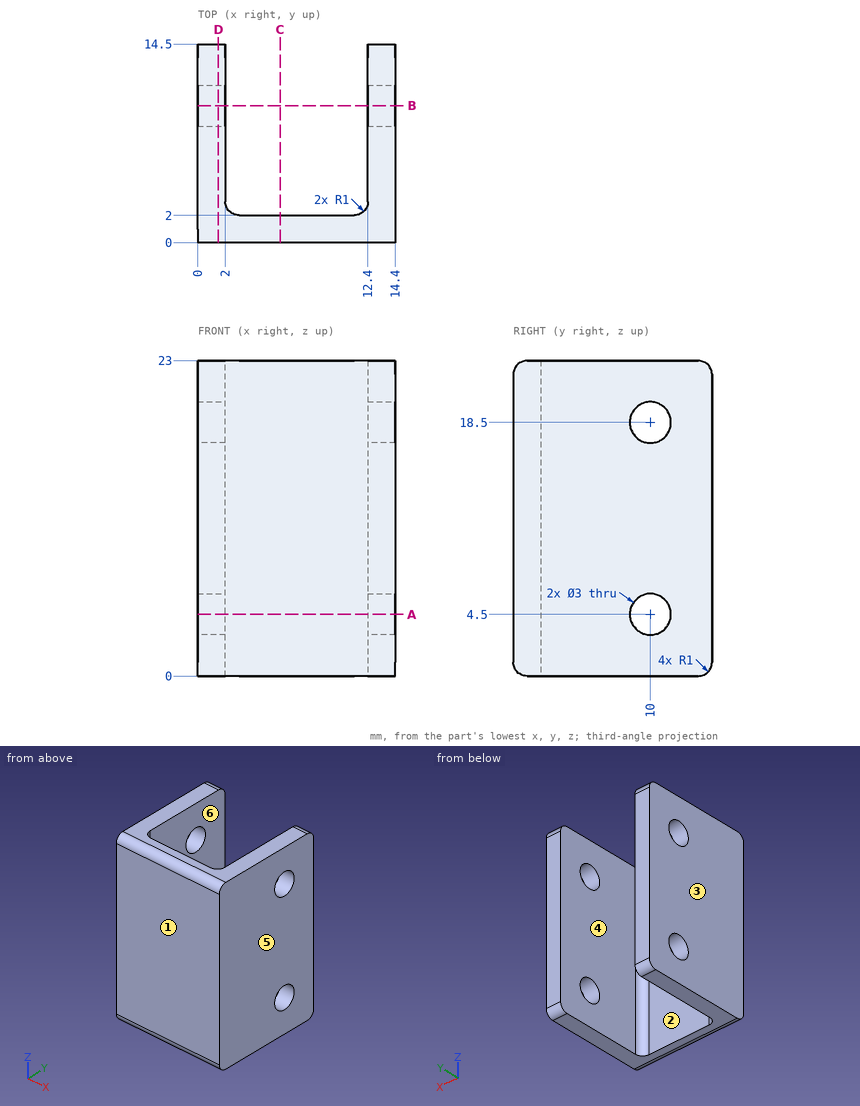
Could you check a few things on this drawing? It's one solid part, dimensions in mm from its lowest x, y, z. A direction names the side the tool comes from. Coordinates: 2 decimals unless noted, no trailing zeros. Order: outer loops, then holes, each group sorted by start corner. A loop starts at its lowest first (then second) coordinate and runs counter-clockwise, first axis right, second up. Notation, with made-up numbers: M 8.25,67.5 L 35.25,67.5 A19 ccw 35.25,101.5 Z; hole C -5.75,-5 d7. An arc over 180 degrees is marked long. Use one line per item in the form item = value. Start each with the question number.
1. Suppose I cut it at D-D on x = 1.5. Write out the boundary of the cut face in (y, z), then the cut area to 3 significant figures.
2. On a 3-axis mill with a long thin cutter (end or side, diameter ignored), from which of +Z, -Z, +X, -X, +Y, -Y can I reach the whole of each face in a straight line? I mean the marked faces 5 and 6. Say none if no direction works.
3. For pin 1 (4 mm diameter, centred on x = 5, y = 12.5, fed in from +Z); pin 2 (5 mm diameter, centred on y = 10, z = 4.5, fed in from -X); pin 3 (2 mm diameter, centred on x = 10.5, z = 12, fed in from +Y) (3 decimals), each with a flat end and sliding along its axis, tell me the tip position at first contact or that it passes through.
4. Please list where these lines run through material, in increasing order: line 1 (X direction, y = 7.25, z = 10.25); line 2 (Y direction, x = 0.4, z = 4.5); line 3 (Y direction, x = 8.25, z = 10.75).
5. We'd pull the mould along X, two halves only. Please class the marked faces 1, 2, 3 and 4: +X half, -X half, draft (parallel to the pull), parting line (faces both ways), or undercut.
6. Suppose I cut it at A-A on z = 4.5. Write out the boundary of the cut face in (x, y), then the cut area to 3 significant figures.
7. Suppose I cut it at C-C on x = 6. Write out the boundary of the cut face in (y, z), then the cut area to 3 significant figures.
8. Suppose I cut it at B-B on y = 10. Write out the boundary of the cut face in (x, z), then the cut area to 3 significant figures.
Geometry says:
q1.outline = M 0,1 A1 ccw 1,0 L 13.5,0 A1 ccw 14.5,1 L 14.5,22 A1 ccw 13.5,23 L 1,23 A1 ccw 0,22 Z; hole C 10,4.5 d3; hole C 10,18.5 d3
q1.area = 319 mm^2
q2.face_5 = +Z, -Z, +X, +Y, -Y
q2.face_6 = +Z, -Z, +Y
q3.pin_1 = through
q3.pin_2 = 0
q3.pin_3 = 2.005
q4.line_1 = 0 to 2, 12.4 to 14.4
q4.line_2 = 0 to 8.5, 11.5 to 14.5
q4.line_3 = 0 to 2
q5.face_1 = draft
q5.face_2 = undercut
q5.face_3 = -X half
q5.face_4 = undercut
q6.outline = M 0,0 L 14.4,0 L 14.4,8.5 L 12.4,8.5 L 12.4,3 A1 cw 11.4,2 L 3,2 A1 cw 2,3 L 2,8.5 L 0,8.5 Z; M 0,11.5 L 2,11.5 L 2,14.5 L 0,14.5 Z; M 12.4,11.5 L 14.4,11.5 L 14.4,14.5 L 12.4,14.5 Z
q6.area = 67.2 mm^2
q7.outline = M 0,1 A1 ccw 1,0 L 2,0 L 2,23 L 1,23 A1 ccw 0,22 Z
q7.area = 45.6 mm^2
q8.outline = M 0,0 L 2,0 L 2,3 L 0,3 Z; M 0,6 L 2,6 L 2,17 L 0,17 Z; M 0,20 L 2,20 L 2,23 L 0,23 Z; M 12.4,0 L 14.4,0 L 14.4,3 L 12.4,3 Z; M 12.4,6 L 14.4,6 L 14.4,17 L 12.4,17 Z; M 12.4,20 L 14.4,20 L 14.4,23 L 12.4,23 Z
q8.area = 68.0 mm^2
